Geometry: final body of the model. Coordinates: model frame, mm. A direction names the side the tool comes from. Coordinates: 2 decimals unless noted, no trailing zeros. Loops run counter-clockwise (first coordinate to the right, second up) from the corner with the lowest first, then second, coordinate; pieces in that order, holes last. Notation, with made-up numbers: (6.25, 50.5) - (53.25, 50.5) arc R18 ccw to (53.25, 61.5) - close; hole circle Ø4 at (10.5, -33.5). An arc over 180 degrees is marked (long way). Answer in a Markdown table with one row per item.
from build123d import *

# Parameters (mm, degrees)
ESQUISSE1_R              = 50
BOSS_EXTRU_1_DEPTH       = 22
ESQUISSE2_R              = 2.5
ENL_V_MAT_EXTRU_1_DEPTH  = 7
ENL_V_START              = -15
ENL_V_MAT_EXTRU_2_DEPTH  = 15
ESQUISSE5_R              = 46.5
ESQUISSE5_R_2            = 6
ENL_V_MAT_EXTRU_3_DEPTH  = 8
ENL_V_START_2            = -8
ESQUISSE7_R              = 46.5
ESQUISSE7_R_2            = 6
ENL_V_MAT_EXTRU_4_DEPTH  = 8
ESQUISSE8_R              = 6
ENL_V_MAT_EXTRU_5_DEPTH  = 8
ESQUISSE9_R              = 6
ENL_V_MAT_EXTRU_6_DEPTH  = 8
ESQUISSE10_R             = 6
ENL_V_MAT_EXTRU_7_DEPTH  = 8
ESQUISSE11_R             = 6
ENL_V_MAT_EXTRU_8_DEPTH  = 8
ESQUISSE12_R             = 6
ENL_V_MAT_EXTRU_10_DEPTH = 8
ESQUISSE13_R             = 6
ENL_V_MAT_EXTRU_11_DEPTH = 8
ESQUISSE14_R             = 6
ENL_V_MAT_EXTRU_12_DEPTH = 8
ESQUISSE15_R             = 6
ENL_V_MAT_EXTRU_13_DEPTH = 8


with BuildPart() as part:
    # Esquisse1 → Boss.-Extru.1 (new body)
    with BuildSketch(Plane.XY):
        Circle(ESQUISSE1_R)
    extrude(amount=BOSS_EXTRU_1_DEPTH)

    # Esquisse2 → Enlèv. mat.-Extru.1 (cut)
    with BuildSketch(Plane.XY.offset(22)):
        Circle(ESQUISSE2_R)
    extrude(amount=-ENL_V_MAT_EXTRU_1_DEPTH, mode=Mode.SUBTRACT)

    # Esquisse4 → Enlèv. mat.-Extru.2 (cut)
    with BuildSketch(Plane(origin=(0, 0, 0), x_dir=(-1, 0, 0), z_dir=(0, 0, -1)).offset(ENL_V_START)):
        with BuildLine():
            ThreePointArc((2.5, 0), (0.887540635, 2.337150321), (-1.869817297, 1.659452704))
            Line((-1.869817297, 1.659452704), (-2.496337165, -0.135280301))
            ThreePointArc((-2.496337165, -0.135280301), (0.06766494, -2.499084123), (2.5, 0))
        make_face()
    extrude(amount=ENL_V_MAT_EXTRU_2_DEPTH, mode=Mode.SUBTRACT)

    # Esquisse5 → Enlèv. mat.-Extru.3 (cut)
    with BuildSketch(Plane(origin=(0, 0, 0), x_dir=(-1, 0, 0), z_dir=(0, 0, -1))):
        Circle(ESQUISSE5_R)
        Circle(ESQUISSE5_R_2, mode=Mode.SUBTRACT)
    extrude(amount=-ENL_V_MAT_EXTRU_3_DEPTH, mode=Mode.SUBTRACT)

    # Esquisse7 → Enlèv. mat.-Extru.4 (cut)
    with BuildSketch(Plane.XY.offset(22).offset(ENL_V_START_2)):
        with Locations(Location((0, 0, 0), (0, 0, 180))):
            Circle(ESQUISSE7_R)
        with Locations(Location((0, 0, 0), (0, 0, 180))):
            Circle(ESQUISSE7_R_2, mode=Mode.SUBTRACT)
    extrude(amount=ENL_V_MAT_EXTRU_4_DEPTH, mode=Mode.SUBTRACT)

    # Esquisse8 → Enlèv. mat.-Extru.5 (cut)
    with BuildSketch(Plane(origin=(0, 0, 8), x_dir=(-1, 0, 0), z_dir=(0, 0, -1))):
        with Locations((-25, 0)):
            Circle(ESQUISSE8_R)
    extrude(amount=-ENL_V_MAT_EXTRU_5_DEPTH, mode=Mode.SUBTRACT)

    # Esquisse9 → Enlèv. mat.-Extru.6 (cut)
    with BuildSketch(Plane(origin=(0, 0, 8), x_dir=(-1, 0, 0), z_dir=(0, 0, -1))):
        with Locations((0, 25)):
            Circle(ESQUISSE9_R)
    extrude(amount=-ENL_V_MAT_EXTRU_6_DEPTH, mode=Mode.SUBTRACT)

    # Esquisse10 → Enlèv. mat.-Extru.7 (cut)
    with BuildSketch(Plane(origin=(0, 0, 8), x_dir=(-1, 0, 0), z_dir=(0, 0, -1))):
        with Locations((25, 0)):
            Circle(ESQUISSE10_R)
    extrude(amount=-ENL_V_MAT_EXTRU_7_DEPTH, mode=Mode.SUBTRACT)

    # Esquisse11 → Enlèv. mat.-Extru.8 (cut)
    with BuildSketch(Plane(origin=(0, 0, 8), x_dir=(-1, 0, 0), z_dir=(0, 0, -1))):
        with Locations((0, -25)):
            Circle(ESQUISSE11_R)
    extrude(amount=-ENL_V_MAT_EXTRU_8_DEPTH, mode=Mode.SUBTRACT)

    # Esquisse12 → Enlèv. mat.-Extru.10 (cut)
    with BuildSketch(Plane(origin=(0, 0, 8), x_dir=(-1, 0, 0), z_dir=(0, 0, -1))):
        with Locations((-17.68, 17.68)):
            Circle(ESQUISSE12_R)
    extrude(amount=-ENL_V_MAT_EXTRU_10_DEPTH, mode=Mode.SUBTRACT)

    # Esquisse13 → Enlèv. mat.-Extru.11 (cut)
    with BuildSketch(Plane(origin=(0, 0, 8), x_dir=(-1, 0, 0), z_dir=(0, 0, -1))):
        with Locations((17.68, 17.68)):
            Circle(ESQUISSE13_R)
    extrude(amount=-ENL_V_MAT_EXTRU_11_DEPTH, mode=Mode.SUBTRACT)

    # Esquisse14 → Enlèv. mat.-Extru.12 (cut)
    with BuildSketch(Plane(origin=(0, 0, 8), x_dir=(-1, 0, 0), z_dir=(0, 0, -1))):
        with Locations((-17.68, -17.68)):
            Circle(ESQUISSE14_R)
    extrude(amount=-ENL_V_MAT_EXTRU_12_DEPTH, mode=Mode.SUBTRACT)

    # Esquisse15 → Enlèv. mat.-Extru.13 (cut)
    with BuildSketch(Plane(origin=(0, 0, 8), x_dir=(-1, 0, 0), z_dir=(0, 0, -1))):
        with Locations((17.68, -17.68)):
            Circle(ESQUISSE15_R)
    extrude(amount=-ENL_V_MAT_EXTRU_13_DEPTH, mode=Mode.SUBTRACT)


solid = part.part
(1) Pull-direction query (X, two-part tool) for faces 4 (the face through (47.69, 15.02, 10.85)), 5 (the face through (33, -33, 22)), 6 (the face through (-5.723, -1.802, 17.944)); classes: pulls with the +X half, pulls with the -X half, needs draft (parallel to the pull), parting line crosses it, or undercut.
Verdict:
| item | result |
|---|---|
| face 4 | parting line crosses it |
| face 5 | needs draft |
| face 6 | undercut |
(2) Cut plane C-C on y = -25. Output: boundary loops of the cut face in (x, z).
Verdict:
| item | result |
|---|---|
| outline | (-43.3, 0) - (-39.21, 0) - (-39.21, 8) - (-6, 8) - (-6, 14) - (-39.21, 14) - (-39.21, 22) - (-43.3, 22) - close; (6, 8) - (39.21, 8) - (39.21, 0) - (43.3, 0) - (43.3, 22) - (39.21, 22) - (39.21, 14) - (6, 14) - close |
(3) Ray query, probe 1 along Y at (x, z) = (0, 10.3); probe 2 along Y at (x, z) = (-17.68, 10.6); probe 3 along Y at (x, z) = (-23, 11.5). Return the intervals inside material, ascending.
Verdict:
| item | result |
|---|---|
| probe 1 | y = -50 to -31, -19 to -2.5, 2.5 to 19, 31 to 50 |
| probe 2 | y = -46.77 to -23.68, -11.68 to 11.68, 23.68 to 46.77 |
| probe 3 | y = -44.4 to -20.45, -14.91 to -5.66, 5.66 to 14.91, 20.45 to 44.4 |
(4) Cut plane D-D on x = -22. Output: boundary loops of the cut face in (y, z).
Verdict:
| item | result |
|---|---|
| outline | (-44.9, 0) - (-40.97, 0) - (-40.97, 8) - (-21.84, 8) - (-21.84, 14) - (-40.97, 14) - (-40.97, 22) - (-44.9, 22) - close; (-13.52, 8) - (-5.2, 8) - (-5.2, 14) - (-13.52, 14) - close; (5.2, 8) - (13.52, 8) - (13.52, 14) - (5.2, 14) - close; (21.84, 8) - (40.97, 8) - (40.97, 0) - (44.9, 0) - (44.9, 22) - (40.97, 22) - (40.97, 14) - (21.84, 14) - close |
(5) Cut plane B-B on x = 4.5. Output: boundary loops of the cut face in (y, z), then the cut area to 3 significant figures.
Verdict:
| item | result |
|---|---|
| outline | (-49.8, 0) - (-46.28, 0) - (-46.28, 8) - (-28.97, 8) - (-28.97, 14) - (-46.28, 14) - (-46.28, 22) - (-49.8, 22) - close; (-21.03, 8) - (-3.97, 8) - (-3.97, 0) - (3.97, 0) - (3.97, 8) - (21.03, 8) - (21.03, 14) - (3.97, 14) - (3.97, 22) - (-3.97, 22) - (-3.97, 14) - (-21.03, 14) - close; (28.97, 8) - (46.28, 8) - (46.28, 0) - (49.8, 0) - (49.8, 22) - (46.28, 22) - (46.28, 14) - (28.97, 14) - close |
| area | 742 mm² |
(6) Access query for faces 1 (the face through (-11.686, -17.416, 10.958)), 2 (the face through (-10, -1, 14)), 3 (the face through (1, -10, 8)). Directions: +Z, -Z, +X, -X, +Y, -Y. A direction counts if a zero-diameter tool reaches every point of the face in a straight line with its end or side. Return the directions, or none.
Verdict:
| item | result |
|---|---|
| face 1 | +Z, -Z |
| face 2 | +Z |
| face 3 | -Z |
(7) First-contact query: pin 1 Ø12 at (y, z) = (-34.5, 3.5) entering from -X; pin 2 Ø14 at (x, y) = (25, 0) entering from -Z; pin 3 Ø0.7 at (x, y) = (2, 0.5) entering from +Z. Flat tips, straight axial feed; report the tip coordinate or a pass-through.
Verdict:
| item | result |
|---|---|
| pin 1 | stops at x = -41.08 |
| pin 2 | stops at z = 8 |
| pin 3 | stops at z = 15 |
(8) Cut plane A-A on z = 4.25. Output: boundary loops of the cut face in (x, y), then the cut area to 3 significant figures.
Verdict:
| item | result |
|---|---|
| outline | circle Ø100 at (0, 0); circle Ø12 at (0, 0); hole circle Ø93 at (0, 0); hole (1.87, 1.66) arc R2.5 ccw (long way) to (2.5, -0.14) - close |
| area | 1,150 mm² |
